Part print with two shaded views. Sizes in mm from the minimum x, y, z corner. A direction names the side the tool comes from. Coordinates: 2 decimals unless noted, no trailing zeros. Loops run counter-clockwise (first coordinate to the right, second up) from the corner with the lowest first, then second, coordinate; pieces in that order, holes last. Notation, with made-up numbers: (44, 65.25) -> (103, 65.25) arc R25 ccw to (103, 91.25) -> close; hole circle Ø8 at (7.5, 85). An arc over 180 degrees is marked (long way). Return JSON: item names as keys, results as strings. Group by question number.
(1) Tool access for the marked faces 1, 2, 3, 4 and 5: list every direction of +Z, -Z, +X, -X, +Y, -Y with a clear straight run to the whole face (end or side of a thin tool).
(2) Flat gauge pins, fed straight in: pin 1 Ø5 at (x, z) = (158.75, 69.87) entering from +Y; pin 2 Ø16.5 at (y, z) = (23, 54) entering from +X; pin 3 Ø12 at (y, z) = (6.5, 48.5) entering from +X; pin 4 Ø12 at (x, y) = (98.5, 4.5) entering from -Z. Where does each tip first touch, or does it go through?
(3) Saw through at B-B on z = 12.7. Write the cut outline in (x, y) (1 decimal).
(4) Saw through at A-A on x = 158.75. Write the cut outline in (y, z) (1 decimal).
(5) Probe L1, parallel to X at y = 5, z = 12.7 (1 decimal); L2, parallel to Z at x = 158.75, y = 22 (1 decimal); L3, parallel to Y at x = 88.5, z = 77.5. List the from-to ranges inside material, lowest first.
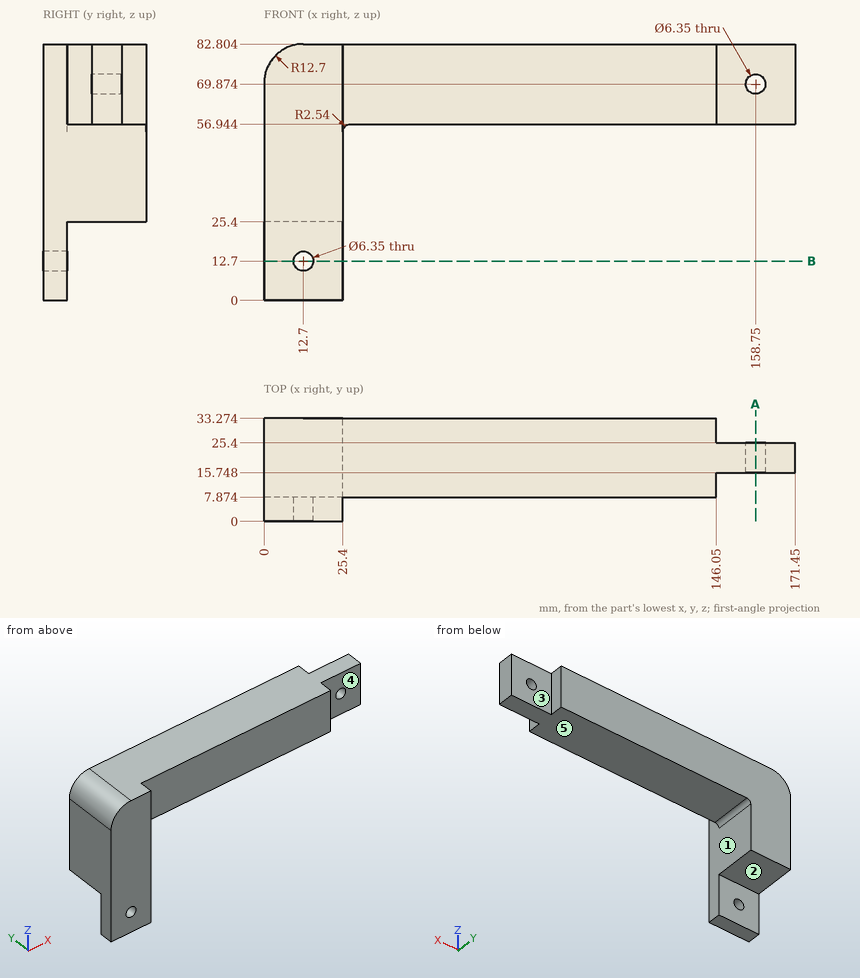
Geometry results:
{
 "1": {"face 1": "-Z, +X, -Y", "face 2": "-Z, +X, -X, +Y", "face 3": "+Z, -Z, +X, +Y", "face 4": "+Z, -Z, +X, -Y", "face 5": "-Z, +X, +Y, -Y"},
 "2": {"pin 1": "through", "pin 2": "x = 171.45", "pin 3": "x = 25.4", "pin 4": "z = 56.94"},
 "3": {"outline": "(0, 0) -> (9.5, 0) -> (9.5, 7.9) -> (0, 7.9) -> close; (15.9, 0) -> (25.4, 0) -> (25.4, 7.9) -> (15.9, 7.9) -> close"},
 "4": {"outline": "(15.7, 56.9) -> (25.4, 56.9) -> (25.4, 66.7) -> (15.7, 66.7) -> close; (15.7, 73) -> (25.4, 73) -> (25.4, 82.8) -> (15.7, 82.8) -> close"},
 "5": {"L1": "0 to 9.5, 15.9 to 25.4", "L2": "56.9 to 66.7, 73 to 82.8", "L3": "7.87 to 33.27"}
}
